The figure shows three views and two pictorial views of one solid part (mm, origin at its lowest corner). Answer the questions. A direction names the side the tool comes from. Give positions to 0.01 mm unless a question says otherwise; leave off trailing zeros. Write each loop counter-clockwise with the first axis right and the second up, starting at its lowest first coordinate (ties: lowest second). Pieces come first, ordered by that corner, then holes. Notation, with made-up numbers: (55, 39) - (107, 39) arc R26 cw to (107, 67) - close; hole circle Ø10 at (9.5, -33). An arc over 180 degrees is marked (long way). Use a Markdown table: item, result. Add a question column.
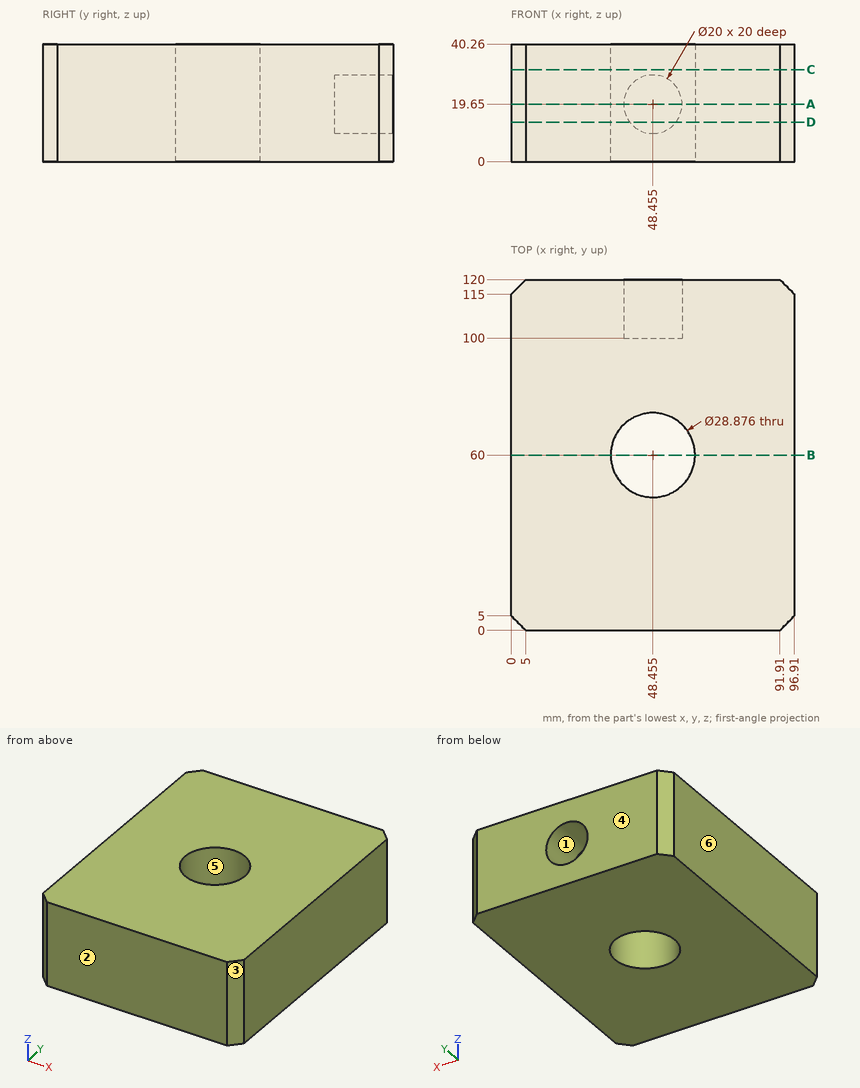
1. The part is cut by section D-D (z = 13.5). Give the vertices of the cut face in (x, y) (1 decimal).
2. For a pull along Y with two mould halves and no side action, classify the marked faces 3, 4, 5 and 6 as released by +Y, released by -Y, zero draft, split by the parting line, or undercut.
3. The part is cut by section A-A (z = 19.65). Give the vertices of the cut face in (x, y) (1 decimal).
4. Given P1, Ø2, axis at x = 83.5, z = 28.5, coming from the -Y side; P2, Ø6, axis at x = 51, z = 15, coming from the +Y side, each flat-ended and moving along its own axis, determine where each tip first touches the part or whether it passes through.
5. The part is cut by section C-C (z = 31.5). Give the vertices of the cut face in (x, y) (1 decimal).
6. The part is cut by section B-B (y = 60). Give the vertices of the cut face in (x, z), and give its area (3 significant figures).
7. Consider L1, parallel to X at y = 105, z = 19.65 (1 decimal); L2, parallel to X at y = 57, z = 14; L3, parallel to Y at x = 54.5, z = 24.5. Determine where each line is inside the solid, lowest interval first. Write a range as [from, to].
8. Which of the six approach directions +Z, -Z, +X, -X, +Y, -Y give full straight-line access (tool end or side, diameter ignored) to the marked faces 1 and 2?
Check values:
| question | item | result |
|---|---|---|
| 1 | outline | (0, 5) - (5, 0) - (91.9, 0) - (96.9, 5) - (96.9, 115) - (91.9, 120) - (56.3, 120) - (56.3, 100) - (40.6, 100) - (40.6, 120) - (5, 120) - (0, 115) - close; hole circle Ø28.9 at (48.5, 60) |
| 2 | face 3 | released by -Y |
| 2 | face 4 | released by +Y |
| 2 | face 5 | undercut |
| 2 | face 6 | zero draft |
| 3 | outline | (0, 5) - (5, 0) - (91.9, 0) - (96.9, 5) - (96.9, 115) - (91.9, 120) - (58.5, 120) - (58.5, 100) - (38.5, 100) - (38.5, 120) - (5, 120) - (0, 115) - close; hole circle Ø28.9 at (48.5, 60) |
| 4 | P1 | stops at y = 0 |
| 4 | P2 | stops at y = 100 |
| 5 | outline | (0, 5) - (5, 0) - (91.9, 0) - (96.9, 5) - (96.9, 115) - (91.9, 120) - (5, 120) - (0, 115) - close; hole circle Ø28.9 at (48.5, 60) |
| 6 | outline | (0, 0) - (34.02, 0) - (34.02, 40.26) - (0, 40.26) - close; (62.89, 0) - (96.91, 0) - (96.91, 40.26) - (62.89, 40.26) - close |
| 6 | area | 2,740 mm2 |
| 7 | L1 | x = [0, 38.5], [58.5, 96.9] |
| 7 | L2 | x = [0, 34.33], [62.58, 96.91] |
| 7 | L3 | y = [0, 46.89], [73.11, 100] |
| 8 | face 1 | +Y |
| 8 | face 2 | +Z, -Z, +X, -X, -Y |
